```python
from build123d import *

# Parameters (mm, degrees)
SKETCH4_W          = 15
SKETCH4_H          = 150
MIDDLE_DEPTH       = 130
SKETCH10_R         = 2
MIDDLE_HOLES_DEPTH = 215.534379529
SKETCH11_W         = 55
SKETCH11_H         = 15
UPPER_DEPTH        = 130
UPPER_START        = 185
UPPER_HOLES_DEPTH  = 15
CUT_EXTRUDE1_DEPTH = 277.631523872


with BuildPart() as part:
    # Sketch4 → Middle (new, symmetric)
    with BuildSketch(Plane(origin=(0, 0, 0), x_dir=(0, 0, -1), z_dir=(1, 0, 0))):
        with Locations((172.5, 95)):
            Rectangle(SKETCH4_W, SKETCH4_H)
    extrude(amount=MIDDLE_DEPTH, both=True)

    # Sketch10 → Middle Holes (cut, through all)
    with BuildSketch(Plane(origin=(0, 0, -180), x_dir=(-1, 0, 0), z_dir=(0, 0, -1))):
        with Locations((-28.5, 150)):
            Circle(SKETCH10_R)
        with Locations((28.5, 150)):
            Circle(SKETCH10_R)
        with Locations((28.5, 73)):
            Circle(SKETCH10_R)
        with Locations((-28.5, 73)):
            Circle(SKETCH10_R)
        with BuildLine():
            Line((-110, 155.7), (-90, 155.7))
            ThreePointArc((-90, 155.7), (-84.3, 150), (-90, 144.3))
            Line((-90, 144.3), (-110, 144.3))
            ThreePointArc((-110, 144.3), (-115.7, 150), (-110, 155.7))
        make_face()
        with BuildLine():
            Line((90, 144.3), (110, 144.3))
            ThreePointArc((110, 144.3), (115.7, 150), (110, 155.7))
            Line((110, 155.7), (90, 155.7))
            ThreePointArc((90, 155.7), (84.3, 150), (90, 144.3))
        make_face()
        with BuildLine():
            Line((-117.7, 60), (-117.7, 40))
            ThreePointArc((-117.7, 40), (-112, 34.3), (-106.3, 40))
            Line((-106.3, 40), (-106.3, 60))
            ThreePointArc((-106.3, 60), (-112, 65.7), (-117.7, 60))
        make_face()
        with BuildLine():
            Line((106.3, 40), (106.3, 60))
            ThreePointArc((106.3, 60), (112, 65.7), (117.7, 60))
            Line((117.7, 60), (117.7, 40))
            ThreePointArc((117.7, 40), (112, 34.3), (106.3, 40))
        make_face()
    extrude(amount=-MIDDLE_HOLES_DEPTH, mode=Mode.SUBTRACT)

    # Sketch11 → Upper (add, symmetric)
    with BuildSketch(Plane(origin=(0, 0, 0), x_dir=(0, 0, -1), z_dir=(1, 0, 0))):
        with Locations((152.5, 177.5)):
            Rectangle(SKETCH11_W, SKETCH11_H)
    extrude(amount=UPPER_DEPTH, both=True)

    # Sketch12 → Upper Holes (cut)
    with BuildSketch(Plane(origin=(0, 0, 0), x_dir=(1, 0, 0), z_dir=(0, 1, 0)).offset(UPPER_START)):
        with BuildLine():
            Line((-110, 139.3), (-90, 139.3))
            ThreePointArc((-90, 139.3), (-84.3, 145), (-90, 150.7))
            Line((-90, 150.7), (-110, 150.7))
            ThreePointArc((-110, 150.7), (-115.7, 145), (-110, 139.3))
        make_face()
        with BuildLine():
            Line((110, 139.3), (90, 139.3))
            ThreePointArc((90, 139.3), (84.3, 145), (90, 150.7))
            Line((90, 150.7), (110, 150.7))
            ThreePointArc((110, 150.7), (115.7, 145), (110, 139.3))
        make_face()
    extrude(amount=-UPPER_HOLES_DEPTH, mode=Mode.SUBTRACT)

    # Sketch14 → Cut-Extrude1 (cut, through all)
    with BuildSketch(Plane(origin=(0, 185, 0), x_dir=(1, 0, 0), z_dir=(0, 1, 0))):
        with BuildLine():
            Line((42.098030274, 145.2), (42.098030274, 146.2))
            ThreePointArc((42.098030274, 146.2), (40.78001079, 149.381980515), (37.598030274, 150.7))
            Line((37.598030274, 150.7), (-7.634483759, 150.7))
            ThreePointArc((-7.634483759, 150.7), (-10.816464274, 149.381980515), (-12.134483759, 146.2))
            Line((-12.134483759, 146.2), (-12.134483759, 145.2))
            ThreePointArc((-12.134483759, 145.2), (-10.816464274, 142.018019485), (-7.634483759, 140.7))
            Line((-7.634483759, 140.7), (37.598030274, 140.7))
            ThreePointArc((37.598030274, 140.7), (40.78001079, 142.018019485), (42.098030274, 145.2))
        make_face()
    extrude(amount=-CUT_EXTRUDE1_DEPTH, mode=Mode.SUBTRACT)


solid = part.part
```
CAD build for the part. Positions are in the model's coordinates, mm. A direction names the side the tool comes from. Round coordinates to 2 decimals unless told otherwise and drop trailing zeros. Write each loop counter-clockwise with the first axis right and the second up, starting at its lowest first coordinate (ties: lowest second). Pieces come first, ordered by that corner, then holes. Notation, with made-up numbers: (72.5, 67) - (113.5, 67) arc R31 cw to (113.5, 91) - close; hole circle Ø8 at (-4.5, -26.75). An arc over 180 degrees is marked (long way). Return JSON: item names as keys, results as strings. Group by question number.
Item 1: Mould opens along Z. For faces 4 (the face through (15, 178, -150.7)), 5 (the face through (2, 101, -180)), 6 (the face through (2, 170, -140)) say: +Z half, -Z half, draft (parallel to the pull), parting line (faces both ways), or undercut.
Item 2: Probe probe 1 along Y at (x, z) = (28.5, -174.25); probe 2 along X at (y, z) = (150, -169); probe 3 along Y at (x, z) = (-103.5, -172). List the from-to ranges inside material, lowest first.
Item 3: Band-saw the part on C-C on y = 100.5. List the corners of the cut face in (x, z), plus the area to 3 significant figures.
Item 4: Flat gauge pin, fed straight in: pin 1 Ø20 at (x, z) = (5.5, -146) entering from -Y. Where does the tip first touch, or does it go through?
Item 5: Band-saw the part on A-A on x = -0.5. List the corners of the cut face in (y, z).
Item 6: Band-saw the part on D-D on z = -133. List the corners of the cut face in (x, y), plus the area to 3 significant figures.
Item 7: 3-axis set-ups, long thin cutter, end or side, ignore diameter. For faces 1 (the face through (-117.7, 50, -173)), 2 (the face through (2, 185, -152)), 3 (the face through (-100, 178, -150.7)): which of +Z, -Z, +X, -X, +Y, -Y reach the whole face in a straight line?
Item 8: Band-saw the part on B-B on x = 69.5. List the corners of the cut face in (y, z), plus the area to 4 significant figures.
Resolved:
{
 "1": {"face 4": "undercut", "face 5": "-Z half", "face 6": "draft"},
 "2": {"probe 1": "y = 20 to 71, 75 to 148, 152 to 185", "probe 2": "x = -130 to -115.7, -84.3 to -30.5, -26.5 to 26.5, 30.5 to 84.3, 115.7 to 130", "probe 3": "y = 20 to 144.3, 155.7 to 185"},
 "3": {"outline": "(-130, -180) - (130, -180) - (130, -165) - (-130, -165) - close", "area": "3,900 mm²"},
 "4": {"pin 1": "stops at y = 170"},
 "5": {"outline": "(20, -180) - (185, -180) - (185, -150.7) - (170, -150.7) - (170, -165) - (20, -165) - close; (170, -140.7) - (185, -140.7) - (185, -125) - (170, -125) - close"},
 "6": {"outline": "(-130, 170) - (130, 170) - (130, 185) - (-130, 185) - close", "area": "3,900 mm²"},
 "7": {"face 1": "+Z, -Z", "face 2": "+Z, -Z, +X, -X, +Y", "face 3": "+Y, -Y"},
 "8": {"outline": "(20, -180) - (185, -180) - (185, -125) - (170, -125) - (170, -165) - (20, -165) - close", "area": "3,075 mm²"}
}
